Design review of the part shown in the three views and the two pictorial views. Dimensions are in mm from the part's minimum x, y and z. Coordinates: 2 decimals unless noted, no trailing zeros. Loops run counter-clockwise (first coordinate to the right, second up) from the corner with the lowest first, then second, coordinate; pieces in that order, holes last. Notation, with made-up numbers: (46, -16) -> (100, -16) arc R15 ccw to (100, -1) -> close; hole circle Ø10 at (21, 44). An arc over 180 degrees is marked (long way). One line per item, written item: value. Start each with the question number.
1. Add section B-B on y = 4. Write out the cut boundary in (x, z).
2. Add section C-C on x = 44.5. Write out the cut boundary in (y, z), plus the area to 3 significant figures.
3. For probe 1 along Y at (x, z) = (10, 0.5); probe 2 along X at (y, z) = (3.5, 0.25), list the stretches that pass through material, from the lowest coordinate up.
4. Add section A-A on x = 10. Write out the cut boundary in (y, z).
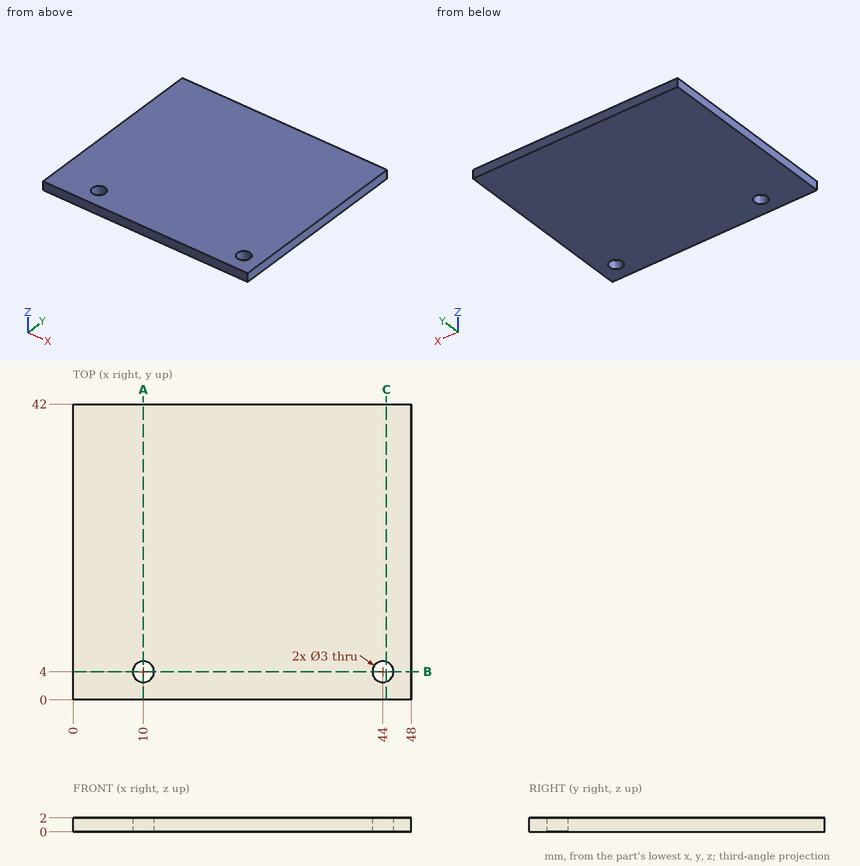
Worked answers:
1. outline: (0, 0) -> (8.5, 0) -> (8.5, 2) -> (0, 2) -> close; (11.5, 0) -> (42.5, 0) -> (42.5, 2) -> (11.5, 2) -> close; (45.5, 0) -> (48, 0) -> (48, 2) -> (45.5, 2) -> close
2. outline: (0, 0) -> (2.59, 0) -> (2.59, 2) -> (0, 2) -> close; (5.41, 0) -> (42, 0) -> (42, 2) -> (5.41, 2) -> close
2. area: 78.3 mm²
3. probe 1: y = 0 to 2.5, 5.5 to 42
3. probe 2: x = 0 to 8.59, 11.41 to 42.59, 45.41 to 48
4. outline: (0, 0) -> (2.5, 0) -> (2.5, 2) -> (0, 2) -> close; (5.5, 0) -> (42, 0) -> (42, 2) -> (5.5, 2) -> close
